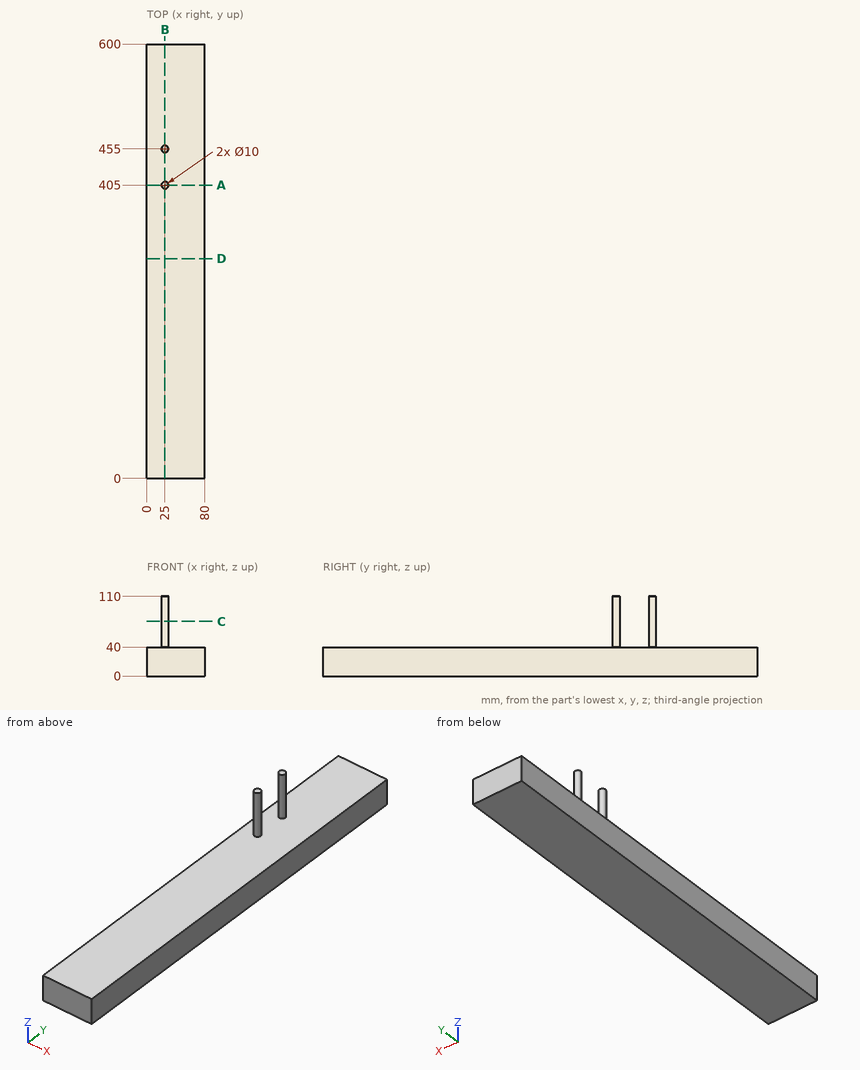
Part print with two shaded views. Sizes in mm from the minimum x, y, z corner. Give positions to 0.01 mm unless a question says otherwise; leave off trailing zeros. Write each loop counter-clockwise with the first axis right and the second up, starting at its lowest first coordinate (ties: lowest second). Pieces come first, ordered by that corner, then holes.
1) Cut at A-A on y = 405. Write the cut outline in (x, z), then the cut area to 3 significant figures.
Resolved:
outline: (0, 0) - (80, 0) - (80, 40) - (30, 40) - (30, 110) - (20, 110) - (20, 40) - (0, 40) - close
area: 3,900 mm2
2) Probe L1, parallel to Y at x = 25.5, z = 45; L2, parallel to Z at x = 63, y = 200. List the from-to ranges inside material, lowest first.
Resolved:
L1: y = 400.03 to 409.97, 450.03 to 459.97
L2: z = 0 to 40
3) Cut at D-D on y = 303.5. Write the cut outline in (x, z).
Resolved:
outline: (0, 0) - (80, 0) - (80, 40) - (0, 40) - close
4) Cut at B-B on x = 25. Write the cut outline in (y, z), then the cut area to 3 significant figures.
Resolved:
outline: (0, 0) - (600, 0) - (600, 40) - (460, 40) - (460, 110) - (450, 110) - (450, 40) - (410, 40) - (410, 110) - (400, 110) - (400, 40) - (0, 40) - close
area: 25,400 mm2
5) Cut at C-C on z = 75.5. Write the cut outline in (x, y).
Resolved:
outline: circle Ø10 at (25, 405); circle Ø10 at (25, 455)
6) Pin check, flat tip, straight feed: pin 1 (8 mm diameter, centred on x = 53.5, y = 498.5, fed in from +Z). Stop position of the tip, or through.
Resolved:
pin 1: stops at z = 40
